Can you work these out from the model? Positions are in its coordinate system, mm. Face numbers are marked on the shaded views. A direction names the side the tool comes from. Round coordinates to 2 decimals unless told otherwise and drop trailing zeros. Order: outer loops, then holes, each group sorted by start corner. A loop starts at its lowest first (then second) coordinate and runs counter-clockwise, first axis right, second up. Notation, with made-up numbers: M -24.75,7.5 L 8.25,7.5 A17 ccw 8.25,27.5 Z; hole C 56.5,83 d1. An arc over 180 degrees is marked long. Answer as a JSON object with one key per item and string values. Group by question number.
Solid Edge part; units mm, degrees
sketch "Sketch1" plane through (0, 0, 0) normal (0, -1, 0) x (1, 0, 0)
  circle A0 centre (0, 0) radius 4
extrude "Protrusion1" add sketch "Sketch1" along normal mid plane 17
sketch "Sketch2" plane through (0, -8.5, 0) normal (0, -1, 0) x (1, 0, 0)
  circle A0 centre (0, 0) radius 3
extrude "ProtrusiónExtruida_2" add sketch "Sketch2" along normal blind 10
chamfer "Chaflán_1" distance 1 angle 45 1 edges at (-3, -18.5, 0)
sketch "Sketch3" plane through (0, 8.5, 0) normal (0, 1, 0) x (0, 0, -1)
  line L0 (3.5, -3.5) -> (-3.5, -3.5)
  line L1 (-3.5, -3.5) -> (-3.5, 3.5)
  line L2 (-3.5, 3.5) -> (3.5, 3.5)
  line L3 (3.5, 3.5) -> (3.5, -3.5)
  line L4 (5, 5) -> (-5, 5)
  line L5 (-5, 5) -> (-5, -5)
  line L6 (-5, -5) -> (5, -5)
  line L7 (5, -5) -> (5, 5)
  dimension "D1" = 3.5
  dimension "D2" = 5
extrude "Cutout1" cut sketch "Sketch3" against normal through all
hole "Agujero_1" at (0, 8.5, 0) direction (0, -1, 0) diameter 5 depth 12 tip angle 82
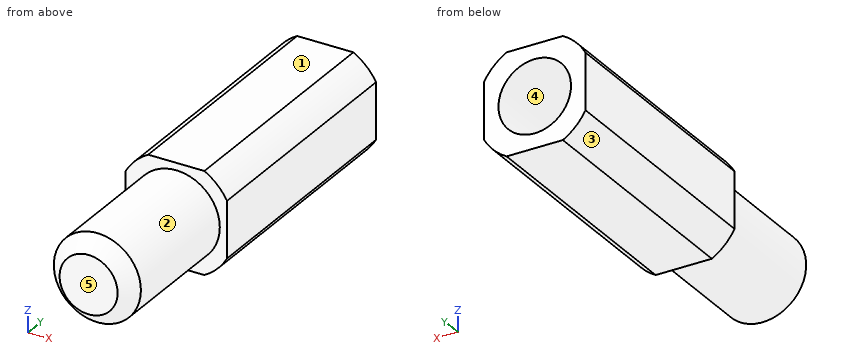
Item 1: Suppose I cut it at D-D, the plane y = -14. Write out the boundary of the cut face in (x, z).
Item 2: I'm going to push a flat-ended pin straight in: pin 1 Ø1.5 at (y, z) = (-10, 2.5) entering from -X. Where does the tip first touch, or does it pass through?
Item 3: If we mould it in two halves opening along Z, with no side actions, what happens to the marked faces 3, 4 and 5? For each: +Z half, -Z half, draft (parallel to the pull), parting line (faces both ways), or undercut.
Item 4: Suppose I cut it at C-C, the plane y = -4.25. Write out the boundary of the cut face in (x, z), and give its area (3 significant figures).
Item 5: On a 3-axis mill with a long thin cutter (end or side, diameter ignored), from which of +Z, -Z, +X, -X, +Y, -Y can I reach the whole of each face in a straight line? I mean the marked faces 1 and 2. Say none if no direction works.
Item 6: I need wall thicknesses on line 1 (X direction, y = 1, z = 0); line 2 (X direction, y = -1, z = 1.5). Which ranges of each line are inside material? Lowest first, please.
Item 7: Suppose I cut it at A-A, the plane y = -0.5. Write out the boundary of the cut face in (x, z), and give its area (3 significant figures).
Item 8: Suppose I cut it at B-B, the plane y = -7. Write out the boundary of the cut face in (x, z).
Computed:
{
 "1": {"outline": "C 0,0 d6"},
 "2": {"pin 1": "stops at x = -2.44"},
 "3": {"face 3": "-Z half", "face 4": "undercut", "face 5": "draft"},
 "4": {"outline": "M -3.5,-1.94 A4 ccw -1.94,-3.5 L 1.94,-3.5 A4 ccw 3.5,-1.94 L 3.5,1.94 A4 ccw 1.94,3.5 L -1.94,3.5 A4 ccw -3.5,1.94 Z; hole C 0,0 d3.7", "area": "34.3 mm^2"},
 "5": {"face 1": "+Z, +X, -X, +Y, -Y", "face 2": "-Y"},
 "6": {"line 1": "x = -3.5 to -2.5, 2.5 to 3.5", "line 2": "x = -3.5 to -2, 2 to 3.5"},
 "7": {"outline": "M -3.5,-1.94 A4 ccw -1.94,-3.5 L 1.94,-3.5 A4 ccw 3.5,-1.94 L 3.5,1.94 A4 ccw 1.94,3.5 L -1.94,3.5 A4 ccw -3.5,1.94 Z; hole C 0,0 d5", "area": "25.4 mm^2"},
 "8": {"outline": "M -3.5,-1.94 A4 ccw -1.94,-3.5 L 1.94,-3.5 A4 ccw 3.5,-1.94 L 3.5,1.94 A4 ccw 1.94,3.5 L -1.94,3.5 A4 ccw -3.5,1.94 Z"}
}
